Read the model definition and answer for the solid it produces. Units are mm, in the model's axes. Face numbers are marked on the shaded views. A direction names the side the tool comes from. Give positions to 0.01 mm unless a question says otherwise; leave off trailing zeros. Write each loop counter-clockwise with the first axis right and the second up, starting at its lowest first coordinate (ties: lowest second). Pieces come first, ordered by that corner, then holes. Notation, with made-up numbers: (29.25, 40) -> (46.25, 40) arc R27 cw to (46.25, 75) -> close; hole circle Ø1 at (11.5, 33.5). An arc over 180 degrees is marked (long way). Use a Markdown table: item, result.
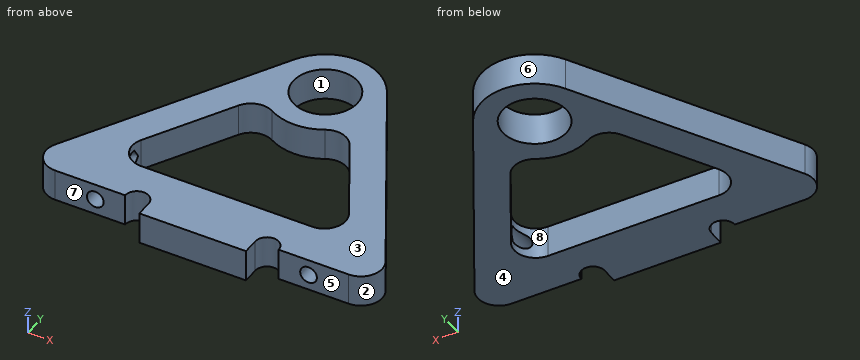
Autodesk Inventor part; units mm, degrees
ref_plane "YZ Plane" through (0, 0, 0) normal (1, 0, 0) x (0, 1, 0)
ref_plane "XZ Plane" through (0, 0, 0) normal (0, 1, 0) x (-1, 0, 0)
ref_plane "XY Plane" through (0, 0, 0) normal (0, 0, 1) x (1, 0, 0)
sketch "スケッチ1" plane through (0, 0, 0) normal (0, 0, 1) x (1, 0, 0)
  circle A0 centre (0, 0) radius 3
  circle A1 centre (0, 0) radius 5
  line L0 (-5, -20) -> (5, -20)
  line L1 (5, -20) -> (5, -21.5)
  line L2 (5, -21.5) -> (-5, -21.5)
  line L3 (-5, -21.5) -> (-5, -20)
  circle A2 centre (-6.1, -20) radius 1.1
  line L4 (0, 0) -> (0, -20) construction
  circle A3 centre (6.1, -20) radius 1.1
  line L5 (-7.2, -20) -> (-17.2, -20)
  line L6 (-17.2, -20) -> (-4.3402, 2.4825)
  line L7 (7.2, -20) -> (17.2, -20)
  line L8 (17.2, -20) -> (4.3402, 2.4825)
  point P0 (0, -21.5)
  point P1 (4.3402, 2.4825)
  dimension "d1" = 10
  dimension "d0" = 6
  dimension "d2" = 10
  dimension "d3" = 1.5
  dimension "d4" = 2.2
  dimension "d5" = 20
  dimension "d6" = 10
extrude "押し出し1" add sketch "スケッチ1" along normal blind 3 contours A1 | A1 L8 L7 A3 L0 A2 L5 L6 | L1 L2 L3 L0
fillet "フィレット1" radius 2 2 edges at (-17.2, -20, 1.5) (17.2, -20, 1.5)
sketch "スケッチ3" plane through (0, 0, 0) normal (0, 0, -1) x (-1, 0, 0)
  arc A0 (-15.488, -17.007) -> (-13.752, -20) centre (-13.752, -18) ccw
  line L0 (-7.2, -20) -> (-13.752, -20)
  arc A1 (-5, -20) -> (-7.2, -20) centre (-6.1, -20) ccw
  line L1 (-5, -21.5) -> (-5, -20)
  line L2 (5, -21.5) -> (-5, -21.5)
  line L3 (5, -20) -> (5, -21.5)
  arc A2 (7.2, -20) -> (5, -20) centre (6.1, -20) ccw
  line L4 (13.752, -20) -> (7.2, -20)
  arc A3 (13.752, -20) -> (15.488, -17.007) centre (13.752, -18) ccw
  line L5 (4.3402, 2.4825) -> (15.488, -17.007)
  arc A4 (4.3402, 2.4825) -> (-4.3402, 2.4825) centre (0, 0) ccw
  line L6 (-15.488, -17.007) -> (-4.3402, 2.4825)
  circle A5 centre (0, 0) radius 3
  line L7 (-11.4559, -16) -> (11.4559, -16)
  line L8 (11.4559, -16) -> (4.0113, -2.9848)
  line L9 (-11.4559, -16) -> (-4.0113, -2.9848)
  line L10 (-15.488, -17.007) -> (-4.3402, 2.4825)
  circle A6 centre (0, 0) radius 5
  line L11 (5, -21.5) -> (-5, -21.5)
  arc A7 (4.3402, 2.4825) -> (-4.3402, 2.4825) centre (0, 0) ccw
  point P0 (0, -21.5)
  point P1 (0, -16)
  point P2 (0, -21.5)
  dimension "d19" = 4
  dimension "d20" = 3
extrude "押し出し2" cut sketch "スケッチ3" against normal through all contours A6 L8 L7 L9
fillet "フィレット2" radius 2 4 edges at (-4.0113, -2.9848, 1.5) (4.0113, -2.9848, 1.5) (-11.4559, -16, 1.5) (11.4559, -16, 1.5)
sketch "スケッチ2" plane through (-17.2, -20, 0) normal (0, -1, 0) x (1, 0, 0)
  line L0 (12.2, 0) -> (12.2, 3)
  line L1 (22.2, 0) -> (22.2, 3)
  point P0 (17.2, 0)
  point P1 (7.2, 1.5)
  point P2 (27.2, 1.5)
  point P3 (12.2, 1.5)
  point P4 (22.2, 1.5)
  point P5 (12.2, 1.5)
  point P6 (22.2, 1.5)
  dimension "d9" = 5
  dimension "d10" = 5
hole "穴1" at (-10, -20, 1.5) at (10, -20, 1.5) direction (0, 1, 0) diameter 1.567 depth 6.3 tip angle 118
sketch "スケッチ4" plane through (0, 0, 0) normal (0, 0, -1) x (-1, 0, 0)
  line L0 (5.405, -15.9) -> (-14.4109, -15.9) construction
  arc A0 (-15.5215, -12.2367) -> (-14.4109, -15.9) centre (-14.4109, -13.9) ccw construction
  line L1 (-15.5215, -12.2367) -> (-4.1487, -4.643) construction
  arc A1 (-2.1701, -4.5045) -> (-4.1487, -4.643) centre (-3.0381, -6.3063) ccw construction
  arc A2 (-2.1701, -4.5045) -> (2.4825, -4.3402) centre (0, 0) ccw construction
  arc A3 (5.2116, -5.0832) -> (2.4825, -4.3402) centre (3.4756, -6.0762) ccw construction
  line L2 (5.2116, -5.0832) -> (7.3308, -8.7882) construction
  arc A4 (7.377, -10.6888) -> (7.3308, -8.7882) centre (5.5948, -9.7812) ccw
  arc A5 (7.377, -10.6888) -> (7.2631, -13.1601) centre (10.0503, -12.0503) ccw
  arc A6 (5.405, -15.9) -> (7.2631, -13.1601) centre (5.405, -13.9) ccw
  line L3 (4.3402, 2.4825) -> (9.529, -6.589) construction
  arc A7 (4.3402, 2.4825) -> (0, 5) centre (0, 0) ccw construction
  line L4 (-8, 5) -> (0, 5) construction
  arc A8 (-8, 5) -> (-10.7765, 4.1583) centre (-8, 0) ccw construction
  line L5 (-33.2416, -10.8417) -> (-10.7765, 4.1583) construction
  arc A9 (-33.2416, -10.8417) -> (-30.4651, -20) centre (-30.4651, -15) ccw construction
  line L6 (-7.2, -20) -> (-30.4651, -20) construction
  arc A10 (-5, -20) -> (-7.2, -20) centre (-6.1, -20) ccw construction
  line L7 (-5, -21.5) -> (-5, -20) construction
  line L8 (5, -21.5) -> (-5, -21.5) construction
  line L9 (5, -20) -> (5, -21.5) construction
  arc A11 (7.2, -20) -> (5, -20) centre (6.1, -20) ccw construction
  line L10 (15, -20) -> (7.2, -20)
  arc A12 (15, -20) -> (17.1213, -19.1213) centre (15, -17) ccw
  line L11 (17.1213, -19.1213) -> (22.0711, -14.1716)
  arc A13 (22.0711, -14.1716) -> (22.0711, -9.9289) centre (19.9497, -12.0503) ccw
  arc A14 (22.0711, -9.9289) -> (11.8876, -7.4967) centre (15, -17) ccw
  arc A15 (9.529, -6.589) -> (11.8876, -7.4967) centre (11.2651, -5.596) ccw
  arc A16 (9.2724, -11.2724) -> (10.8281, -12.8281) centre (10.0503, -12.0503) ccw
  arc A17 (20.7276, -11.2724) -> (9.2724, -11.2724) centre (15, -17) ccw
  arc A18 (19.1719, -12.8281) -> (20.7276, -11.2724) centre (19.9497, -12.0503) ccw
  arc A19 (19.1719, -12.8281) -> (10.8281, -12.8281) centre (15, -17) ccw
  line L12 (-9.6659, 2.495) -> (-32.131, -12.505) construction
  arc A20 (-6.3341, -2.495) -> (-9.6659, 2.495) centre (-8, 0) ccw construction
  line L13 (-28.7992, -17.495) -> (-6.3341, -2.495) construction
  arc A21 (-32.131, -12.505) -> (-28.7992, -17.495) centre (-30.4651, -15) ccw construction
  circle A22 centre (0, 0) radius 3 construction
  circle A23 centre (15, -17) radius 1.1
  line L14 (5.405, -15.9) -> (5.405, -16)
  line L15 (8.0079, -16) -> (-8.0079, -16)
  arc A24 (-2.4825, -4.3402) -> (2.4825, -4.3402) centre (0, 0) ccw
  arc A25 (5.2116, -5.0832) -> (2.4825, -4.3402) centre (3.4756, -6.0762) ccw
  line L16 (5.2116, -5.0832) -> (9.744, -13.007)
  arc A26 (8.0079, -16) -> (9.744, -13.007) centre (8.0079, -14) ccw
  line L17 (8.0079, -16) -> (-8.0079, -16)
  arc A27 (-9.744, -13.007) -> (-8.0079, -16) centre (-8.0079, -14) ccw
  line L18 (-9.744, -13.007) -> (-5.2116, -5.0832)
  arc A28 (-2.4825, -4.3402) -> (-5.2116, -5.0832) centre (-3.4756, -6.0762) ccw
  arc A29 (-15.488, -17.007) -> (-13.752, -20) centre (-13.752, -18) ccw
  line L19 (-7.2, -20) -> (-13.752, -20)
  arc A30 (-5, -20) -> (-7.2, -20) centre (-6.1, -20) ccw
  line L20 (-5, -21.5) -> (-5, -20)
  line L21 (5, -21.5) -> (-5, -21.5)
  line L22 (5, -20) -> (5, -21.5)
  arc A31 (7.2, -20) -> (5, -20) centre (6.1, -20) ccw
  line L23 (13.752, -20) -> (7.2, -20)
  arc A32 (13.752, -20) -> (15.488, -17.007) centre (13.752, -18) ccw
  line L24 (4.3402, 2.4825) -> (15.488, -17.007)
  arc A33 (4.3402, 2.4825) -> (-4.3402, 2.4825) centre (0, 0) ccw
  line L25 (-15.488, -17.007) -> (-4.3402, 2.4825)
  circle A34 centre (0, 0) radius 3
  point P0 (9.529, -6.589)
  point P1 (11.3484, -9.7698)
  point P2 (12.4427, -11.683)
  point P3 (14.86, -15.909)
  point P4 (15.743, -17.8111)
  point P5 (9.8052, -13.1226)
  point P6 (9.0034, -11.7124)
  point P7 (7.3308, -8.7882)
sketch "スケッチ5" plane through (0, 0, 0) normal (0, 0, -1) x (-1, 0, 0)
  circle A0 centre (15, -17) radius 2
  arc A1 (20.7276, -11.2724) -> (9.2724, -11.2724) centre (15, -17) ccw
  arc A2 (9.2724, -11.2724) -> (10.8281, -12.8281) centre (10.0503, -12.0503) ccw
  arc A3 (19.1719, -12.8281) -> (10.8281, -12.8281) centre (15, -17) ccw
  arc A4 (19.1719, -12.8281) -> (20.7276, -11.2724) centre (19.9497, -12.0503) ccw
  arc A5 (18.5355, -13.4645) -> (11.4645, -13.4645) centre (15, -17) ccw
  arc A6 (8.636, -10.636) -> (11.4645, -13.4645) centre (10.0503, -12.0503) ccw
  arc A7 (21.364, -10.636) -> (8.636, -10.636) centre (15, -17) ccw
  arc A8 (18.5355, -13.4645) -> (21.364, -10.636) centre (19.9497, -12.0503) ccw
  point P0 (0, 0)
properties part number "kosipiti" material "アルミニウム 2014-T4"
Item 1: A cutting plane is placed at D-D (x = 12.5). Give the vertices of the cut face in (y, z), then the cut area to 3 significant figures.
Return value:
| item | result |
|---|---|
| outline | (-20, 0) -> (-11.78, 0) -> (-11.78, 3) -> (-20, 3) -> close |
| area | 24.7 mm^2 |
Item 2: A cutting plane is placed at B-B (x = 1). Give the vertices of the cut face in (y, z), then the cut area to 3 significant figures.
Return value:
| item | result |
|---|---|
| outline | (-21.5, 0) -> (-16, 0) -> (-16, 3) -> (-21.5, 3) -> close; (-4.9, 0) -> (-2.83, 0) -> (-2.83, 3) -> (-4.9, 3) -> close; (2.83, 0) -> (4.9, 0) -> (4.9, 3) -> (2.83, 3) -> close |
| area | 28.9 mm^2 |
Item 3: Straight lines are drawn through the part: line 1 along Y through (x, z) = (0, 0.3); line 2 along Y through (x, z) = (2.5, 0.25); line 3 along Z through (x, y) = (-10, -15). For each, find the intervals that lie inside material, in ascending order. Write a range as [from, to].
Return value:
| item | result |
|---|---|
| line 1 | [-21.5, -16], [-5, -3], [3, 5] |
| line 2 | [-21.5, -16], [-4.33, -1.66], [1.66, 4.33] |
| line 3 | [0, 0.72], [2.28, 3] |
Item 4: A cutting plane is placed at C-C (y = -8). Give the vertices of the cut face in (x, z).
Return value:
| item | result |
|---|---|
| outline | (-10.34, 0) -> (-6.88, 0) -> (-6.88, 3) -> (-10.34, 3) -> close; (6.88, 0) -> (10.34, 0) -> (10.34, 3) -> (6.88, 3) -> close |
Item 5: A tool of negligible diameter and unlimited length cuts with its end or side. For the marked faces 4, 5, 6, 7 and 8, from which of +Z, -Z, +X, -X, +Y, -Y can it reach the whole face along a straight path? Write none if from no direction.
Return value:
| item | result |
|---|---|
| face 4 | -Z, +X, -X, +Y, -Y |
| face 5 | +Z, -Z, +X, -Y |
| face 6 | +Z, -Z, +Y |
| face 7 | +Z, -Z, -X, -Y |
| face 8 | +Z, -Z |
Item 6: Each of these flat-tipped pins is pushed along its axis until it touches: P1, Ø1.8, axis at x = 10, z = 1.5, coming from the +Y side; P2, Ø1, axis at x = 9, z = 2.5, coming from the -Y side; P3, Ø1.5, axis at y = -19, z = 1.5, coming from the -X side; P4, Ø5, axis at x = -5.5, y = -18.5, coming from the -Z side. Where does it stop, or does it pass through?
Return value:
| item | result |
|---|---|
| P1 | y = -5.84 |
| P2 | y = -20 |
| P3 | x = -15.74 |
| P4 | z = 0 |
Item 7: For a pull along Y with two mould halves and no side action, classify the marked faces 1, 2 and 3 as +Y half, -Y half, draft (parallel to the pull), parting line (faces both ways), or undercut.
Return value:
| item | result |
|---|---|
| face 1 | undercut |
| face 2 | parting line |
| face 3 | draft |
Item 8: A cutting plane is placed at A-A (y = -0.5). Give the vertices of the cut face in (x, z), then the cut area to 3 significant figures.
Return value:
| item | result |
|---|---|
| outline | (-6.05, 0) -> (-2.96, 0) -> (-2.96, 3) -> (-6.05, 3) -> close; (2.96, 0) -> (6.05, 0) -> (6.05, 3) -> (2.96, 3) -> close |
| area | 18.5 mm^2 |
